from build123d import *

# Parameters (mm, degrees)
SKETCH_1_R      = 5
EXTRUDE_1_DEPTH = 17
CHAMFER_1_SIZE  = 1
CHAMFER_1_SIZE2 = 0.953570685


# Read off the part's stored shape, not the designer's step: 3/8-16 机械螺纹 螺柱1
with BuildPart() as part:
    # 草图1 → 凸台-拉伸1 (new body)
    with BuildSketch(Plane.XY):
        Circle(SKETCH_1_R)
    extrude(amount=-EXTRUDE_1_DEPTH)

    # 3/8-16 机械螺纹 螺柱1 outline → 3/8-16 机械螺纹 螺柱1 (revolve, cut)
    with BuildSketch(Plane.XZ):
        Polygon((5, 0), (3.81635, 0), (4.7625, -0.94615), (4.7625, -17), (5, -17), align=None)
    revolve(axis=Axis((0, 0, 0), (0, 0, 1)), mode=Mode.SUBTRACT)

    # 草图4 → 旋转1 (revolve)
    with BuildSketch(Plane(origin=(0, 0, 0), x_dir=(0, 0, -1), z_dir=(1, 0, 0)), mode=Mode.PRIVATE) as revolve_1_sk:
        Polygon((17, 0), (37.344329095, 0), (63, 0), (63, 9.3), (17, 7), align=None)
    revolve(revolve_1_sk.sketch.rotate(Axis((0, 0, -37.344329095), (0, 0, -1)), 270), axis=Axis((0, 0, -37.344329095), (0, 0, -1)))

    # 倒角1
    chamfer_1_edges = [part.edges().sort_by_distance(p)[0] for p in [
        (9.3, 0, -63),
    ]]
    chamfer_1_side = [part.faces().sort_by_distance(p)[0] for p in [
        (0, 0, -63),
    ]]
    chamfer(chamfer_1_edges, length=CHAMFER_1_SIZE, length2=CHAMFER_1_SIZE2, reference=chamfer_1_side[0])


solid = part.part
Geometry check sheet. Reference: the model listing, model coordinates, mm. A direction names the side the tool comes from. Round coordinates to 2 decimals unless told otherwise and drop trailing zeros. Loops run counter-clockwise (first coordinate to the right, second up) from the corner with the lowest first, then second, coordinate; pieces in that order, holes last. Notation, with made-up numbers: (57.5, 26) - (106.5, 26) arc R24 ccw to (106.5, 54) - close; hole circle Ø4 at (31, -25). An arc over 180 degrees is marked (long way). Answer as CSV lines item,"result".
(1) Cross-section at A-A, the plane y = 0. Enter the section's corners in (x, z).
Output values:
outline,"(-9.25, -62.05) - (-8.3, -63) - (8.3, -63) - (9.25, -62.05) - (7, -17) - (4.76, -17) - (4.76, -0.95) - (3.82, 0) - (-3.82, 0) - (-4.76, -0.95) - (-4.76, -17) - (-7, -17) - close"
(2) Set-up check for faces 1 (the face through (-1, -5, -17)), 2 (the face through (0, 0, -63)): record each of +Z, -Z, +X, -X, +Y, -Y from which the full face is reachable in a straight line by a thin tool's end or side.
Output values:
face 1,"+Z"
face 2,"-Z, +X, -X, +Y, -Y"
(3) Cross-section at C-C, the plane z = -35. Enter the section's corners in (x, y).
Output values:
outline,"circle Ø15.8 at (0, 0)"
(4) Depth check by flat-ended pin: pin 1 Ø6 at (x, z) = (-6.5, -10) entering from -Y; pin 2 Ø2 at (x, z) = (0, -41) entering from -Y; pin 3 Ø2 at (x, y) = (4.5, 4) entering from +Z. Enter the tip coordinate at first touch or a pass-through.
Output values:
pin 1,"stops at y = -3.23"
pin 2,"stops at y = -8.25"
pin 3,"stops at z = -17"
(5) Material ranges on line 1 along Z through (x, y) = (-1.5, -6.75); line 2 along Y through (x, z) = (5.75, -54.5); line 3 along Y through (x, z) = (0.5, -11), recorded low to high.
Output values:
line 1,"z = -63 to -17"
line 2,"y = -6.76 to 6.76"
line 3,"y = -4.74 to 4.74"
(6) Cross-section at D-D, the plane z = -14.5. Enter the section's corners in (x, y) (1 decimal).
Output values:
outline,"circle Ø9.5 at (0, 0)"
